Autodesk Inventor part; units mm, degrees
ref_plane "YZ Plane" through (0, 0, 0) normal (1, 0, 0) x (0, 1, 0)
ref_plane "XZ Plane" through (0, 0, 0) normal (0, 1, 0) x (-1, 0, 0)
ref_plane "XY Plane" through (0, 0, 0) normal (0, 0, 1) x (1, 0, 0)
sketch "Boceto1" plane through (0, 0, 0) normal (0, 0, 1) x (1, 0, 0)
  line L0 (0, 0) -> (0, 100)
  line L1 (80, 55) -> (83, 55)
  line L2 (83, 55) -> (83, 25)
  line L3 (83, 25) -> (80, 25)
  line L4 (80, 70) -> (80, 55)
  line L5 (80, 25) -> (80, 0)
  line L6 (10, 100) -> (10, 103)
  line L7 (10, 103) -> (40, 103)
  line L8 (40, 103) -> (40, 100)
  line L9 (0, 100) -> (10, 100)
  line L10 (40, 100) -> (68, 100)
  line L11 (77, 75.5) -> (68, 75.5)
  line L12 (68, 75.5) -> (68, 100)
  line L13 (10, 0) -> (10, -3)
  line L14 (40, -3) -> (40, 0)
  line L15 (10, -3) -> (40, -3)
  line L16 (80, 0) -> (40, 0)
  line L17 (10, 0) -> (0, 0)
  line L18 (80, 70) -> (77, 70)
  line L19 (77, 70) -> (77, 75.5)
  point P0 (0, 0)
  dimension "d5" = 30
  dimension "d9" = 30
  dimension "d11" = 10
  dimension "d13" = 3
  dimension "d16" = 80
  dimension "d17" = 3
  dimension "d22" = 3
  dimension "d23" = 100
  dimension "d24" = 25
  dimension "d26" = 3
  dimension "d29" = 9
  dimension "d30" = 70
  dimension "d31" = 75.5
extrude "Extrusión1" add sketch "Boceto1" along normal blind 3
properties part number "Celda pared divisora"
Geometry check sheet. Reference: the model listing, model coordinates, mm. A direction names the side the tool comes from. Coordinates: 2 decimals unless noted, no trailing zeros. Loops run counter-clockwise (first coordinate to the right, second up) from the corner with the lowest first, then second, coordinate; pieces in that order, holes last. Notation, with made-up numbers: (8, 8) - (54, 8) arc R4 cw to (54, 15) - close; hole circle Ø8 at (19, 16). An arc over 180 degrees is marked (long way). Use one line per item in the form item = value. Start each with the question number.
Item 1: Section check C-C, the plane x = 70. Enter the section's corners in (y, z), and give its area (4 significant figures).
Item 2: Thickness scan on probe 1 along Y at (x, z) = (76, 0.85); probe 2 along X at (y, z) = (64.5, 1.5); probe 3 along Y at (x, z) = (79.5, 1.6). Record the ranges inside material, lowest first.
Item 3: Gauge pin test, flat ends, axial feed: pin 1 (1.5 mm diameter, centred on y = 101, z = 2, fed in from +X); pin 2 (0.9 mm diameter, centred on y = 13.5, z = 1, fed in from +X); pin 3 (6 mm diameter, centred on x = 56, y = 35.5, fed in from -Z); pin 4 (1.5 mm diameter, centred on x = 79, z = 1.5, fed in from +Y). Record the tip position at first contact, or that the pin passes through.
Item 4: Section check B-B, the plane y = 15.5. Enter the section's corners in (x, z).
Item 5: Tool access check on faces 1 (the face through (79, 70, 1)), 2 (the face through (10, -1, 1)), 3 (the face through (10, 101, 1)), 4 (the face through (40, -2, 1)). Record the directions out of +Z, -Z, +X, -X, +Y, -Y that give a thin tool (end or side, any length) a straight path to the whole face; none if there is none.
Item 6: Section check A-A, the plane z = 0.45. Enter the section's corners in (x, y).
Computed:
q1.outline = (0, 0) - (75.5, 0) - (75.5, 3) - (0, 3) - close
q1.area = 226.5 mm2
q2.probe_1 = 0 to 75.5
q2.probe_2 = 0 to 80
q2.probe_3 = 0 to 70
q3.pin_1 = 40
q3.pin_2 = 80
q3.pin_3 = 0
q3.pin_4 = 70
q4.outline = (0, 0) - (80, 0) - (80, 3) - (0, 3) - close
q5.face_1 = +Z, -Z, +X, +Y
q5.face_2 = +Z, -Z, -X, -Y
q5.face_3 = +Z, -Z, -X, +Y
q5.face_4 = +Z, -Z, +X, -Y
q6.outline = (0, 0) - (10, 0) - (10, -3) - (40, -3) - (40, 0) - (80, 0) - (80, 25) - (83, 25) - (83, 55) - (80, 55) - (80, 70) - (77, 70) - (77, 75.5) - (68, 75.5) - (68, 100) - (40, 100) - (40, 103) - (10, 103) - (10, 100) - (0, 100) - close
